Autodesk Inventor part; units mm, degrees
ref_plane "Work Plane1" through (0, 0, 8) normal (0, 0, 1) x (1, 0, 0)
ref_plane "YZ Plane" through (0, 0, 0) normal (1, 0, 0) x (0, 1, 0)
ref_plane "XZ Plane" through (0, 0, 0) normal (0, 1, 0) x (-1, 0, 0)
sketch "Sketch2" plane through (0, 0, 0) normal (0, 0, 1) x (1, 0, 0)
  circle A0 centre (0, 0) radius 4
  circle A1 centre (0, 0) radius 7.5
  dimension "d0" = 8
  dimension "d1" = 15
extrude "Extrusion1" add sketch "Sketch2" along normal blind 16
ref_plane "Work Plane1" through (0, 0, 8) normal (0, 0, 1) x (1, 0, 0)
sketch "Sketch3" plane through (0, 0, 8) normal (0, 0, 1) x (1, 0, 0)
  circle A0 centre (0, 0) radius 6.5
  circle A1 centre (0, 0) radius 8
  circle A2 centre (0, 0) radius 4
  dimension "d4" = 13
  dimension "d5" = 16
  dimension "d6" = 8
extrude "Extrusion2" cut sketch "Sketch3" along normal mid plane 3 contours A1
chamfer "Chamfer1" distance 0.25 angle 45 2 edges at (-7.5, 0, 16) (-7.5, 0, 0)
chamfer "Chamfer2" distance 0.75 angle 45 2 edges at (-4, 0, 16) (-4, 0, 0)
chamfer "Chamfer3" distance 0.25 angle 45 2 edges at (-7.5, 0, 9.5) (-7.5, 0, 6.5)
properties part number "Striped Bushing" material "Brass, Soft Yellow"
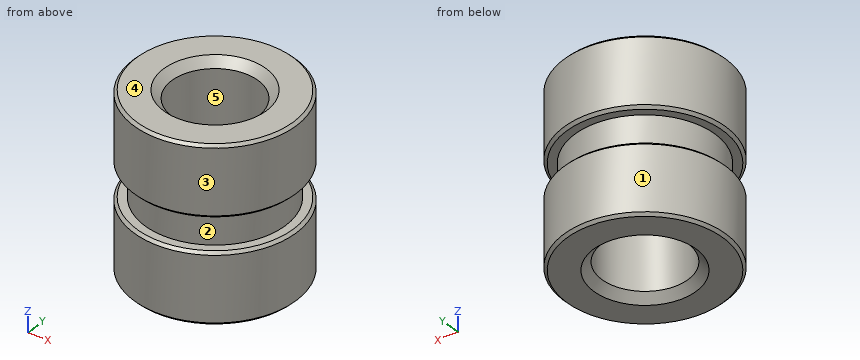
Input: part model. Units: mm. Frame: model coordinates. Face numbers are marked on the shaded views. A direction names the side the tool comes from. Round coordinates to 2 decimals unless told otherwise and drop trailing zeros. Loops run counter-clockwise (first coordinate to the right, second up) from the corner with the lowest first, then second, coordinate; pieces in that order, holes last. Notation, with made-up numbers: (53, 48.25) -> (102, 48.25) arc R24 ccw to (102, 72.25) -> close; hole circle Ø10 at (-18.75, 22.25). An arc over 180 degrees is marked (long way). Use one line per item in the form item = value. Start each with the question number.
Item 1: Mould query, pull axis X, two halves, no side actions, for the marked faces 3, 4 and 5. Classes: pulls with the +X half, pulls with the -X half, needs draft (parallel to the pull), parting line crosses it, or undercut.
Item 2: Material intervals for L1, parallel to Y at x = 0, z = 9.25; L2, parallel to Y at x = 0, z = 11.5; L3, parallel to Z at x = 4, y = 5.75, sorted ascending. Write a range as from..to.
Item 3: Section query C-C on z = 3.25. Return the cut outline in (x, y).
Item 4: Section query A-A on y = 0. Return the cut outline in (x, z), then the cut area to 3 significant figures.
Item 5: Set-up query: the marked faces 1 and 2. Return all of +Z, -Z, +X, -X, +Y, -Y with unobstructed straight access to the full face (end or side cutting, diameter ignored); none if empty.
Item 6: Contact query for flat-ended pins moving along their axis: pin 1 Ø3 at (y, z) = (-3, 9.5) entering from +X; pin 2 Ø1.5 at (x, z) = (4, 13) entering from +Y; pin 3 Ø5 at (y, z) = (-6, 6.5) entering from +X. Output: stop coordinate, or through.
Ans:
q1.face_3 = parting line crosses it
q1.face_4 = needs draft
q1.face_5 = undercut
q2.L1 = -6.5..-4, 4..6.5
q2.L2 = -7.5..-4, 4..7.5
q2.L3 = 0..6.5, 9.5..16
q3.outline = circle Ø15 at (0, 0); hole circle Ø8 at (0, 0)
q4.outline = (-7.5, 0.25) -> (-7.25, 0) -> (-4.75, 0) -> (-4, 0.75) -> (-4, 15.25) -> (-4.75, 16) -> (-7.25, 16) -> (-7.5, 15.75) -> (-7.5, 9.75) -> (-7.25, 9.5) -> (-6.5, 9.5) -> (-6.5, 6.5) -> (-7.25, 6.5) -> (-7.5, 6.25) -> close; (4, 0.75) -> (4.75, 0) -> (7.25, 0) -> (7.5, 0.25) -> (7.5, 6.25) -> (7.25, 6.5) -> (6.5, 6.5) -> (6.5, 9.5) -> (7.25, 9.5) -> (7.5, 9.75) -> (7.5, 15.75) -> (7.25, 16) -> (4.75, 16) -> (4, 15.25) -> close
q4.area = 105 mm^2
q5.face_1 = +Z, -Z
q5.face_2 = none
q6.pin_1 = 7.34
q6.pin_2 = 6.76
q6.pin_3 = 6.63
